Model file for the job. Use its own axes, mm. Give positions to 0.01 mm unless a question says otherwise; leave off trailing zeros. Write each loop counter-clockwise with the first axis right and the second up, starting at its lowest first coordinate (ties: lowest second). Pieces come first, ordered by that corner, then holes. Notation, with made-up numbers: (48.25, 86.5) - (53.25, 86.5) arc R9 ccw to (53.25, 95.5) - close; hole circle Ø11 at (24.25, -36.75). An arc over 180 degrees is marked (long way). Use CSV: the item, a comma, the result in double quotes.
from build123d import *

# Parameters (mm, degrees)
SKETCH1_W               = 4
SKETCH1_H               = 5
BOSS_EXTRUDE1_DEPTH     = 1.75
FILLET1_R               = 0.2
SKETCH3_W               = 0.4
SKETCH3_H               = 0.1
LPATTERN1_COUNT         = 4
LPATTERN1_PITCH         = 1.2
MIRROR1_COPY_1_SKETCH_W = 0.4
MIRROR1_COPY_1_SKETCH_H = 0.1
MIRROR1_COPY_2_SKETCH_W = 0.4
MIRROR1_COPY_2_SKETCH_H = 0.1
MIRROR1_COPY_3_SKETCH_W = 0.4
MIRROR1_COPY_3_SKETCH_H = 0.1


with BuildPart() as part:
    # Sketch1 → Boss-Extrude1 (new body)
    with BuildSketch(Plane(origin=(0, 0, 0), x_dir=(1, 0, 0), z_dir=(0, 1, 0))):
        Rectangle(SKETCH1_W, SKETCH1_H)
    extrude(amount=BOSS_EXTRUDE1_DEPTH)

    # Fillet1
    fillet1_edges = [part.edges().sort_by_distance(p)[0] for p in [
        (-2, 1.75, 0),
        (0, 1.75, 2.5),
        (2, 1.75, 0),
        (0, 0, 2.5),
        (-2, 0, 0),
        (0, 0, -2.5),
        (2, 0, 0),
        (0, 1.75, -2.5),
    ]]
    fillet(fillet1_edges, radius=FILLET1_R)

    # Sweep1: sweep along a path in Sketch2
    with BuildLine(Plane(origin=(0, 0, -1.8), x_dir=(-1, 0, 0), z_dir=(0, 0, -1))) as sweep1_path:
        Line((2, 0.875), (2.3, 0.875))
        ThreePointArc((2.3, 0.875), (2.441421356, 0.816421356), (2.5, 0.675))
        Line((2.5, 0.675), (2.5, 0.25))
        ThreePointArc((2.5, 0.25), (2.558578644, 0.108578644), (2.7, 0.05))
        Line((2.7, 0.05), (3.2, 0.05))
    # Sketch3 → Sweep1 (sweep)
    with BuildSketch(Plane.ZY.offset(2)):
        with Locations((-1.8, 0.875)):
            Rectangle(SKETCH3_W, SKETCH3_H)
    sweep1 = sweep(path=sweep1_path.line)

    # LPattern1: Sweep1 ×4
    with Locations(*[(0, 0, i * LPATTERN1_PITCH) for i in range(1, LPATTERN1_COUNT)]):
        add(sweep1)

    # Mirror1: Sweep1 across plane
    add(sweep1.mirror(Plane(origin=(0, 0, 0), x_dir=(0, 0, 1), z_dir=(1, 0, 0))))

    # Mirror1 copy 1: sweep along a path in Mirror1 copy 1 path
    with BuildLine(Plane(origin=(0, 0, -0.6), x_dir=(1, 0, 0), z_dir=(0, 0, -1))) as mirror1_copy_1_path:
        Line((2, -0.875), (2.3, -0.875))
        ThreePointArc((2.3, -0.875), (2.441421356, -0.816421356), (2.5, -0.675))
        Line((2.5, -0.675), (2.5, -0.25))
        ThreePointArc((2.5, -0.25), (2.558578644, -0.108578644), (2.7, -0.05))
        Line((2.7, -0.05), (3.2, -0.05))
    # Mirror1 copy 1 sketch → Mirror1 copy 1 (sweep)
    with BuildSketch(Plane(origin=(2, 0, 1.2), x_dir=(0, 0, 1), z_dir=(1, 0, 0))):
        with Locations((-1.8, -0.875)):
            Rectangle(MIRROR1_COPY_1_SKETCH_W, MIRROR1_COPY_1_SKETCH_H)
    sweep(path=mirror1_copy_1_path.line)

    # Mirror1 copy 2: sweep along a path in Mirror1 copy 2 path
    with BuildLine(Plane(origin=(0, 0, 0.6), x_dir=(1, 0, 0), z_dir=(0, 0, -1))) as mirror1_copy_2_path:
        Line((2, -0.875), (2.3, -0.875))
        ThreePointArc((2.3, -0.875), (2.441421356, -0.816421356), (2.5, -0.675))
        Line((2.5, -0.675), (2.5, -0.25))
        ThreePointArc((2.5, -0.25), (2.558578644, -0.108578644), (2.7, -0.05))
        Line((2.7, -0.05), (3.2, -0.05))
    # Mirror1 copy 2 sketch → Mirror1 copy 2 (sweep)
    with BuildSketch(Plane(origin=(2, 0, 2.4), x_dir=(0, 0, 1), z_dir=(1, 0, 0))):
        with Locations((-1.8, -0.875)):
            Rectangle(MIRROR1_COPY_2_SKETCH_W, MIRROR1_COPY_2_SKETCH_H)
    sweep(path=mirror1_copy_2_path.line)

    # Mirror1 copy 3: sweep along a path in Mirror1 copy 3 path
    with BuildLine(Plane(origin=(0, 0, 1.8), x_dir=(1, 0, 0), z_dir=(0, 0, -1))) as mirror1_copy_3_path:
        Line((2, -0.875), (2.3, -0.875))
        ThreePointArc((2.3, -0.875), (2.441421356, -0.816421356), (2.5, -0.675))
        Line((2.5, -0.675), (2.5, -0.25))
        ThreePointArc((2.5, -0.25), (2.558578644, -0.108578644), (2.7, -0.05))
        Line((2.7, -0.05), (3.2, -0.05))
    # Mirror1 copy 3 sketch → Mirror1 copy 3 (sweep)
    with BuildSketch(Plane(origin=(2, 0, 3.6), x_dir=(0, 0, 1), z_dir=(1, 0, 0))):
        with Locations((-1.8, -0.875)):
            Rectangle(MIRROR1_COPY_3_SKETCH_W, MIRROR1_COPY_3_SKETCH_H)
    sweep(path=mirror1_copy_3_path.line)


solid = part.part
(1) Saw through at D-D, the plane z = 1.35. List the corners of the cut face in (x, y), then the cut area to 3 significant figures.
Checked values:
outline,"(-2, 0.2) arc R0.2 ccw to (-1.8, 0) - (1.8, 0) arc R0.2 ccw to (2, 0.2) - (2, 1.55) arc R0.2 ccw to (1.8, 1.75) - (-1.8, 1.75) arc R0.2 ccw to (-2, 1.55) - close"
area,"6.97 mm^2"
(2) Saw through at C-C, the plane y = 1. List the corners of the cut face in (x, z), then the cut area to 3 significant figures.
Checked values:
outline,"(-2, -2.5) - (2, -2.5) - (2, 2.5) - (-2, 2.5) - close"
area,"20.0 mm^2"
(3) Wall check: probe 1 along X at (y, z) = (1.5, -0.85); probe 2 along Z at (x, y) = (0.5, 0.15). Give the ranges that are in metal, low to high. Write a range as [from, to].
Checked values:
probe 1,"x = [-2, 2]"
probe 2,"z = [-2.49, 2.49]"
(4) Saw through at A-A, the plane y = 0.35. Count the separate pieces of the cut face and the enclosed holes in it, then the cut area to 3 significant figures.
Checked values:
separate pieces,"9"
enclosed holes,"0"
area,"20.3 mm^2"
(5) Flat gauge pins, fed straight in: P1, Ø0.7, axis at x = 2.5, y = 0.5, coming from the -Z side; P2, Ø0.7, axis at x = 3, y = 0.5, coming from the -Z side. Where does each tip first touch, or does it go through?
Checked values:
P1,"stops at z = -2"
P2,"passes through"
